Build history of the part. All positions in model axes, mm. Give positions to 0.01 mm unless a question says otherwise; leave off trailing zeros. Order: outer loops, then holes, each group sorted by start corner. A loop starts at its lowest first (then second) coordinate and runs counter-clockwise, first axis right, second up. Notation, with made-up numbers: (87, 40) -> (91, 40) arc R24 ccw to (91, 74) -> close; hole circle Ø8 at (-6.75, 12). An arc over 180 degrees is marked (long way). One line per question, with ' | ' between items. Start each with the question number.
(1) Cut at A-A (z = -9.5). Give the cut face in (x, y).
(2) Cut at C-C (x = -29). Give the cut face in (y, z).
(3) Cut at B-B (y = -1.15). Give the cut face in (x, z), then the cut area to 3 significant figures.
(4) Drill centre lines: L1, parallel to Z at x = -14, y = 0.5; L2, parallel to Z at x = -95.5, y = 1.3; L3, parallel to X at y = -0.3, z = 15. Where is each one in solid material? Low to high. Write a range as from..to.
(5) Pin check, flat tips, straight feed: pin 1 Ø6 at (x, z) = (-23.5, -19) entering from +Y; pin 2 Ø1.5 at (x, y) = (-56, -1.5) entering from -Z. Stop position of each tip, or through.
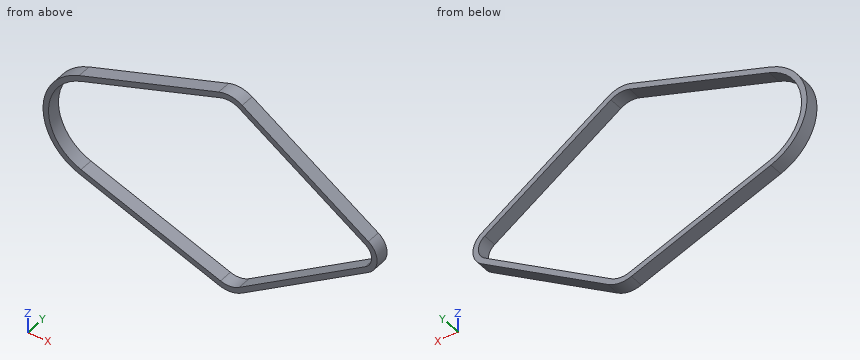
Autodesk Inventor part; units mm, degrees
ref_plane "YZ Plane" through (0, 0, 0) normal (1, 0, 0) x (0, 1, 0)
ref_plane "XZ Plane" through (0, 0, 0) normal (0, 1, 0) x (-1, 0, 0)
ref_plane "XY Plane" through (0, 0, 0) normal (0, 0, 1) x (1, 0, 0)
sketch "Sketch1" plane through (0, 0, 0) normal (0, 1, 0) x (-1, 0, 0)
  arc A0 (-3.2626, 5.0354) -> (-3.2626, -5.0354) centre (0, 0) ccw
  line L0 (0, 0) -> (47.5, 0) construction
  line L1 (47.5, 0) -> (47.5, -27.5) construction
  line L2 (47.5, 0) -> (47.5, 27.5) construction
  arc A1 (42.742, -34.8433) -> (50.4234, -35.7472) centre (47.5, -27.5) ccw
  arc A2 (50.4234, 35.7472) -> (42.742, 34.8433) centre (47.5, 27.5) ccw
  line L3 (47.5, 0) -> (95, 0) construction
  arc A3 (101.2811, -17.7197) -> (101.2811, 17.7197) centre (95, 0) ccw
  line L4 (101.2811, 17.7197) -> (50.4234, 35.7472)
  line L5 (101.2811, -17.7197) -> (50.4234, -35.7472)
  line L6 (42.742, -34.8433) -> (-3.2626, -5.0354)
  line L7 (42.742, 34.8433) -> (-3.2626, 5.0354)
  dimension "d0" = 12
  dimension "d1" = 47.5
  dimension "d2" = 27.5
  dimension "d3" = 27.5
  dimension "d4" = 17.5
  dimension "d5" = 17.5
  dimension "d6" = 47.5
  dimension "d7" = 37.6
sketch "Sketch2" plane through (0, 0, 0) normal (0, 0, 1) x (1, 0, 0)
  line L0 (0, 0) -> (6, 0)
  line L1 (5, 2.5) -> (5, -2.5)
  line L2 (5, -2.5) -> (7, -2.5)
  line L3 (7, -2.5) -> (7, 2.5)
  line L4 (7, 2.5) -> (5, 2.5)
  line L5 (5, 2.5) -> (7, -2.5) construction
  line L6 (5, -2.5) -> (7, 2.5) construction
  dimension "d8" = 6
  dimension "d9" = 2
  dimension "d10" = 5
sweep "Sweep1" add profiles "Sketch2" path "Sketch1"
properties part number "GT2_TimingBelt Base" material "Rubber"
Result set:
1) outline: (-112.37, -2.5) -> (-110.05, -2.5) -> (-110.05, 2.5) -> (-112.37, 2.5) -> close; (-5.47, -2.5) -> (-1.79, -2.5) -> (-1.79, 2.5) -> (-5.47, 2.5) -> close
2) outline: (-2.5, -27.13) -> (2.5, -27.13) -> (2.5, -24.75) -> (-2.5, -24.75) -> close; (-2.5, 24.75) -> (2.5, 24.75) -> (2.5, 27.13) -> (-2.5, 27.13) -> close
3) outline: (-101.62, -18.66) -> (-50.76, -36.69) arc R9.75 ccw to (-42.2, -35.68) -> (3.81, -5.87) arc R7 ccw to (3.81, 5.87) -> (-42.2, 35.68) arc R9.75 ccw to (-50.76, 36.69) -> (-101.62, 18.66) arc R19.8 ccw to start; hole (-100.95, -16.78) -> (-50.09, -34.8) arc R7.75 ccw to (-43.29, -34) -> (2.72, -4.2) arc R5 ccw to (2.72, 4.2) -> (-43.29, 34) arc R7.75 ccw to (-50.09, 34.8) -> (-100.95, 16.78) arc R17.8 ccw to start | area: 584 mm2
4) L1: z = -17.41..-15.03, 15.03..17.41 | L2: z = -20.83..-18.71, 18.71..20.83 | L3: x = -107.92..-104.58, -13.96..-10.28
5) pin 1: stops at y = 2.5 | pin 2: stops at z = -35.1
